```python
from build123d import *

# Parameters (mm, degrees)
SKETCH1_R           = 1.905
SKETCH1_W           = 70.15200002
SKETCH1_H           = 140.473361982
BOSS_EXTRUDE1_DEPTH = 2
BOSS_EXTRUDE2_DEPTH = 4


with BuildPart() as part:
    # Sketch1 → Boss-Extrude1 (new body)
    with BuildSketch(Plane(origin=(0, 0, 0), x_dir=(1, 0, 0), z_dir=(0, 1, 0))):
        Polygon((-19.149417529, -87.154200597), (-19.149417529, 56.047080778), (-27.25676908, 64.16156963), (-90.194065977, 64.16156963), (-98.301422703, 56.047100861), (-98.301422703, -87.154180513), (-90.194058216, -95.261534652), (-27.256776842, -95.261534652), align=None)
        with Locations((-85.141420182, -88.451514751)):
            Circle(SKETCH1_R, mode=Mode.SUBTRACT)
        with Locations((-32.309420182, -88.451514751)):
            Circle(SKETCH1_R, mode=Mode.SUBTRACT)
        with Locations((-32.309420182, 57.344485249)):
            Circle(SKETCH1_R, mode=Mode.SUBTRACT)
        with Locations((-85.141420182, 57.344485249)):
            Circle(SKETCH1_R, mode=Mode.SUBTRACT)
        with Locations((-58.725420192, -15.553513417)):
            Rectangle(SKETCH1_W, SKETCH1_H, mode=Mode.SUBTRACT)
    extrude(amount=BOSS_EXTRUDE1_DEPTH)

    # Sketch1_3 → Boss-Extrude2 (add)
    with BuildSketch(Plane(origin=(0, 0, 0), x_dir=(1, 0, 0), z_dir=(0, 1, 0))):
        Polygon((-27.25676908, 64.16156963), (-90.194065977, 64.16156963), (-98.301422703, 56.047100861), (-98.301422703, -87.154180513), (-90.194058216, -95.261534652), (-27.256776842, -95.261534652), (-19.149417529, -87.154200597), (-19.149417529, 56.047080778), align=None)
        Polygon((-88.951438098, 61.154505914), (-95.301420183, 54.804485249), (-95.301420183, -85.911514751), (-88.951420183, -92.261514751), (-28.499420182, -92.261514751), (-22.14941613, -85.911557384), (-22.14941613, 54.804442616), (-28.499624487, 61.154505914), align=None, mode=Mode.SUBTRACT)
    extrude(amount=BOSS_EXTRUDE2_DEPTH)


solid = part.part
```
Model file for the job. Use its own axes, mm. A direction names the side the tool comes from. Coordinates: 2 decimals unless noted, no trailing zeros. Order: outer loops, then holes, each group sorted by start corner. A loop starts at its lowest first (then second) coordinate and runs counter-clockwise, first axis right, second up. Notation, with made-up numbers: (-19, 22) -> (26, 22) arc R16 ccw to (26, 48) -> close; hole circle Ø11 at (19, 65). An arc over 180 degrees is marked (long way). Return JSON: item names as keys, results as strings.
Item 1: Pin check, flat tip, straight feed: P1, Ø4.5, axis at x = -32.31, z = 88.45, coming from the +Y side. Stop position of the tip, or through.
Model answer:
{"P1": "stops at y = 2"}
Item 2: 3-axis set-ups, long thin cutter, end or side, ignore diameter. For faces 1 (the face through (-25.28, 2.986, -57.935)), 2 (the face through (-83.38, 0.99, 89.18)): which of +Z, -Z, +X, -X, +Y, -Y reach the whole face in a straight line?
Model answer:
{"face 1": "+Y", "face 2": "+Y, -Y"}
Item 3: Slice it at C-C (y = 3.35). Write the cut outline in (x, z).
Model answer:
{"outline": "(-98.3, -56.05) -> (-90.19, -64.16) -> (-27.26, -64.16) -> (-19.15, -56.05) -> (-19.15, 87.15) -> (-27.26, 95.26) -> (-90.19, 95.26) -> (-98.3, 87.15) -> close; hole (-95.3, -54.8) -> (-88.95, -61.15) -> (-28.5, -61.15) -> (-22.15, -54.8) -> (-22.15, 85.91) -> (-28.5, 92.26) -> (-88.95, 92.26) -> (-95.3, 85.91) -> close"}
Item 4: Mould opens along Z. For faces 3 (the face through (-23.1, 2, -60)), 4 (the face through (-92.082, 2.986, -58.024)), 5 (the face through (-23.26, 1.972, 91.265)) say: pulls with the +Z half, pulls with the -Z half, needs draft (parallel to the pull), parting line crosses it, or undercut.
Model answer:
{"face 3": "pulls with the -Z half", "face 4": "undercut", "face 5": "pulls with the +Z half"}
Item 5: Slice it at B-B (x = -51). Write the cut outline in (y, z).
Model answer:
{"outline": "(0, -64.16) -> (4, -64.16) -> (4, -61.15) -> (2, -61.15) -> (2, -54.68) -> (0, -54.68) -> close; (0, 85.79) -> (2, 85.79) -> (2, 92.26) -> (4, 92.26) -> (4, 95.26) -> (0, 95.26) -> close"}
Item 6: Slice it at A-A (z = 75). Write the cut outline in (x, y), then the cut area to 3 significant figures.
Model answer:
{"outline": "(-98.3, 0) -> (-93.8, 0) -> (-93.8, 2) -> (-95.3, 2) -> (-95.3, 4) -> (-98.3, 4) -> close; (-23.65, 0) -> (-19.15, 0) -> (-19.15, 4) -> (-22.15, 4) -> (-22.15, 2) -> (-23.65, 2) -> close", "area": "30.0 mm²"}
Item 7: Wall check: line 1 along X through (y, z) = (1.9, 29.5); line 2 along X through (y, z) = (3.4, 26); line 3 along Z through (x, y) = (-36, 3.7). Give the ranges that are in metal, low to high. Write a range as from..to.
Model answer:
{"line 1": "x = -98.3..-93.8, -23.65..-19.15", "line 2": "x = -98.3..-95.3, -22.15..-19.15", "line 3": "z = -64.16..-61.15, 92.26..95.26"}
